from build123d import *

# Parameters (mm, degrees)
F0_W     = 736.6
F0_H     = 304.8
F1_DEPTH = 44.45
F3_DEPTH = 736.601
F5_DEPTH = 304.801


with BuildPart() as f1:
    # F0 (on Front) → F1 (new body)
    with BuildSketch(Plane.XZ):
        with Locations((294.213133, 152.4)):
            Rectangle(F0_W, F0_H)
    extrude(amount=F1_DEPTH)

    # F2 (on face) → F3 (cut, through all)
    with BuildSketch(Plane.YZ.offset(662.513133)):
        Polygon((-44.45, 101.6), (-12.7, 304.8), (-82.839599, 304.8), (-82.839599, 0), (-12.7, 0), align=None)
    extrude(amount=-F3_DEPTH, mode=Mode.SUBTRACT)

    # F4 (on face) → F5 (cut, through all)
    with BuildSketch(Plane(origin=(0, 0, 0), x_dir=(1, 0, 0), z_dir=(0, 0, -1))):
        Polygon((662.513133, 0), (662.513133, 50.8), (611.713133, 0), align=None)
        Polygon((-23.286867, 0), (-74.086867, 50.8), (-74.086867, 0), align=None)
    extrude(amount=-F5_DEPTH, mode=Mode.SUBTRACT)


solid = f1.part
CAD build for the part. Positions are in the model's coordinates, mm. Give positions to 0.01 mm unless a question says otherwise; leave off trailing zeros. Order: outer loops, then holes, each group sorted by start corner. A loop starts at its lowest first (then second) coordinate and runs counter-clockwise, first axis right, second up. Notation, with made-up numbers: (-38.75, -23) - (-5.75, -23) arc R25 cw to (-5.75, 1) - close; hole circle Ø9 at (-7.75, -8.5). An arc over 180 degrees is marked (long way). Answer in a Markdown table with one row per item.
1. Saw through at B-B, the plane z = 118. Give the cut face in (x, y), plus the area to 3 significant figures.
Data:
| item | result |
|---|---|
| outline | (-65.17, -41.89) - (653.6, -41.89) - (611.71, 0) - (-23.29, 0) - close |
| area | 28,400 mm² |
2. Saw through at C-C, the plane y = -30.5. Give the cut face in (x, z), plus the area to 3 significant figures.
Data:
| item | result |
|---|---|
| outline | (-53.79, 56.96) - (642.21, 56.96) - (642.21, 190.88) - (-53.79, 190.88) - close |
| area | 93,200 mm² |
3. Saw through at A-A, the plane x = 108. Give the cut face in (y, z), plus the area to 3 significant figures.
Data:
| item | result |
|---|---|
| outline | (-44.45, 101.6) - (-12.7, 0) - (0, 0) - (0, 304.8) - (-12.7, 304.8) - close |
| area | 8,710 mm² |
4. Probe probe 1 along Y at (x, z) = (210, 180); probe 2 along Y at (x, z) = (83, 43); probe 3 along X at (y, z) = (-33, 143.5). List the from-to ranges inside material, lowest first. Write a range as [from, to].
Data:
| item | result |
|---|---|
| probe 1 | y = [-32.2, 0] |
| probe 2 | y = [-26.14, 0] |
| probe 3 | x = [-56.29, 644.71] |
5. Flat gauge pins, fed straight in: pin 1 (8 mm diameter, centred on x = 313, z = 148.5, fed in from -Y); pin 2 (1.5 mm diameter, centred on y = -25.5, z = 71.5, fed in from +X); pin 3 (10 mm diameter, centred on x = 556.5, z = 224.5, fed in from -Y); pin 4 (8 mm diameter, centred on y = -29, z = 34.5, fed in from +X). Where does each tip first touch, or does it go through?
Data:
| item | result |
|---|---|
| pin 1 | stops at y = -37.75 |
| pin 2 | stops at x = 637.96 |
| pin 3 | stops at y = -26.03 |
| pin 4 | passes through |
